from build123d import *

# Parameters (mm, degrees)
SKETCH1_W               = 25.4
SKETCH1_H               = 25.4
BOSS_EXTRUDE1_DEPTH     = 25.4
SKETCH2_W               = 22.4536
SKETCH2_H               = 20.447
CUT_EXTRUDE1_DEPTH      = 25.055020349
CUT_EXTRUDE2_DEPTH      = 32.108519733
CUT_EXTRUDE2_DEPTH_BACK = 32.108519733
SKETCH3_R               = 8.89
SKETCH4_R               = 63.5
SKETCH4_R_2             = 11.43
CUT_EXTRUDE3_DEPTH      = 26.814448745
FILLET1_R               = 1.27
FILLET2_R               = 1.27
FILLET3_R               = 0.254


with BuildPart() as part:
    # Sketch1 → Boss-Extrude1 (new body)
    with BuildSketch(Plane.XY):
        Rectangle(SKETCH1_W, SKETCH1_H)
    extrude(amount=-BOSS_EXTRUDE1_DEPTH)

    # Sketch2 → Cut-Extrude1 (cut, through all)
    with BuildSketch(Plane.XY.offset(-9.398)):
        Rectangle(SKETCH2_W, SKETCH2_H)
    extrude(amount=-CUT_EXTRUDE1_DEPTH, mode=Mode.SUBTRACT)

    # Sketch3 → Cut-Extrude2 (cut, two sides: drawn at the far end of the back side and taken through both)
    with BuildSketch(Plane.XY.offset(-CUT_EXTRUDE2_DEPTH_BACK)):
        Circle(SKETCH3_R)
    extrude(amount=CUT_EXTRUDE2_DEPTH + CUT_EXTRUDE2_DEPTH_BACK, mode=Mode.SUBTRACT)

    # Sketch4 → Cut-Extrude3 (cut, through all)
    with BuildSketch(Plane.XY.offset(-6.858)):
        Circle(SKETCH4_R)
        Circle(SKETCH4_R_2, mode=Mode.SUBTRACT)
    extrude(amount=CUT_EXTRUDE3_DEPTH, mode=Mode.SUBTRACT)

    # Fillet1
    fillet1_edges = [part.edges().sort_by_distance(p)[0] for p in [
        (-11.2268, 0, -9.398),
        (0, -10.2235, -9.398),
        (11.2268, 0, -9.398),
        (0, 10.2235, -9.398),
    ]]
    fillet(fillet1_edges, radius=FILLET1_R)

    # Fillet2
    # the kernel refuses this fillet: 1.27 mm, written as the material it adds along each edge
    with BuildSketch(Plane(origin=(-9.9568, 8.9535, -10.668), x_dir=(-1, 0, 0), z_dir=(0, 1, 0))) as fillet2_piece_1_section:
        Polygon((0, 0), (FILLET2_R, 0), (FILLET2_R, FILLET2_R), (0, FILLET2_R), align=None)
    fillet2_piece_1 = extrude(amount=FILLET2_R, mode=Mode.PRIVATE)
    fillet2_piece_1 = fillet2_piece_1 - Plane(origin=(-9.9568, 8.9535, -10.668), x_dir=(0.7071067811865475, 0, -0.7071067811865475), z_dir=(0, 1, 0)) * Sphere(FILLET2_R, mode=Mode.PRIVATE)
    add(fillet2_piece_1)
    with BuildSketch(Plane(origin=(9.9568, 8.9535, -10.668), x_dir=(0, 1, 0), z_dir=(1, 0, 0))) as fillet2_piece_2_section:
        Polygon((0, 0), (FILLET2_R, 0), (FILLET2_R, FILLET2_R), (0, FILLET2_R), align=None)
    fillet2_piece_2 = extrude(amount=FILLET2_R, mode=Mode.PRIVATE)
    fillet2_piece_2 = fillet2_piece_2 - Plane(origin=(9.9568, 8.9535, -10.668), x_dir=(0, -0.7071067811865475, -0.7071067811865475), z_dir=(1, 0, 0)) * Sphere(FILLET2_R, mode=Mode.PRIVATE)
    add(fillet2_piece_2)
    with BuildSketch(Plane(origin=(-9.9568, -8.9535, -10.668), x_dir=(-1, 0, 0), z_dir=(0, -1, 0))) as fillet2_piece_3_section:
        Polygon((0, 0), (FILLET2_R, 0), (FILLET2_R, -FILLET2_R), (0, -FILLET2_R), align=None)
    fillet2_piece_3 = extrude(amount=FILLET2_R, mode=Mode.PRIVATE)
    fillet2_piece_3 = fillet2_piece_3 - Plane(origin=(-9.9568, -8.9535, -10.668), x_dir=(0.7071067811865475, 0, -0.7071067811865475), z_dir=(0, -1, 0)) * Sphere(FILLET2_R, mode=Mode.PRIVATE)
    add(fillet2_piece_3)
    with BuildSketch(Plane(origin=(9.9568, -8.9535, -10.668), x_dir=(0, -1, 0), z_dir=(1, 0, 0))) as fillet2_piece_4_section:
        Polygon((0, 0), (FILLET2_R, 0), (FILLET2_R, -FILLET2_R), (0, -FILLET2_R), align=None)
    fillet2_piece_4 = extrude(amount=FILLET2_R, mode=Mode.PRIVATE)
    fillet2_piece_4 = fillet2_piece_4 - Plane(origin=(9.9568, -8.9535, -10.668), x_dir=(0, 0.7071067811865475, -0.7071067811865475), z_dir=(1, 0, 0)) * Sphere(FILLET2_R, mode=Mode.PRIVATE)
    add(fillet2_piece_4)
    with BuildSketch(Plane(origin=(-11.2268, -10.2235, -10.668), x_dir=(1, 0, 0), z_dir=(0, 0, -1)), Plane(origin=(11.2268, -10.2235, -10.668), x_dir=(0, 1, 0), z_dir=(0, 0, -1))) as fillet2_piece_5:
        with BuildLine():
            CenterArc((FILLET2_R, -FILLET2_R), FILLET2_R, 90, 90)
            Line((0, -FILLET2_R), (0, 0))
            Line((0, 0), (FILLET2_R, 0))
        make_face()
    extrude(amount=14.732)
    with BuildSketch(Plane(origin=(-11.2268, 10.2235, -10.668), x_dir=(1, 0, 0), z_dir=(0, 0, -1)), Plane(origin=(11.2268, 10.2235, -10.668), x_dir=(0, -1, 0), z_dir=(0, 0, -1))) as fillet2_piece_6:
        with BuildLine():
            CenterArc((FILLET2_R, FILLET2_R), FILLET2_R, 180, 90)
            Line((0, FILLET2_R), (0, 0))
            Line((0, 0), (FILLET2_R, 0))
        make_face()
    extrude(amount=14.732)

    # Fillet3
    fillet3_edges = [part.edges().sort_by_distance(p)[0] for p in [
        (-8.89, 0, 0),
        (-8.89, 0, -9.398),
    ]]
    fillet(fillet3_edges, radius=FILLET3_R)


solid = part.part
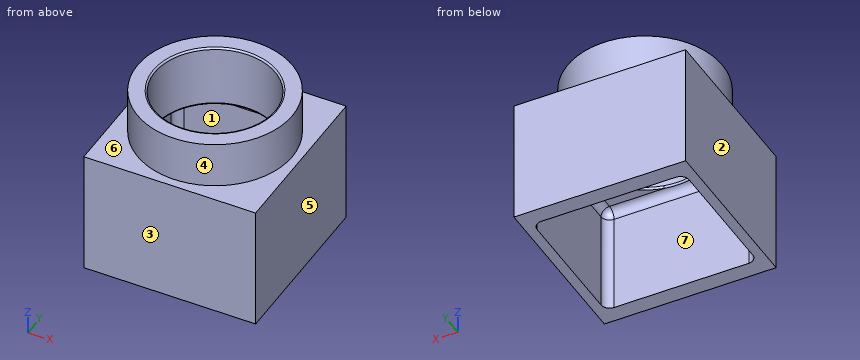
Read the model definition and answer for the solid it produces. Units are mm, in the model's axes. Face numbers are marked on the shaded views. A direction names the side the tool comes from. Coordinates: 2 decimals unless noted, no trailing zeros. Loops run counter-clockwise (first coordinate to the right, second up) from the corner with the lowest first, then second, coordinate; pieces in that order, holes last.
Q1. The part is cut by section C-C on x = 10.75. Write down the section's boundary in (y, z).
Q2. Consider probe 1 along Y at (x, z) = (0, -3.75); probe 2 along Y at (x, z) = (5.75, -18). Determine where each line is inside the solid, lowest interval first.
Q3. The part is cut by section D-D on z = -6.5. Write down the section's boundary in (x, y).
Q4. The part is cut by section A-A on y = 0. Write down the section's boundary in (x, z), and give its area (3 significant figures).
Q5. The part is cut by section B-B on z = -16.5. Write down the section's boundary in (x, y).
Q6. Each of these flat-tipped pins is pushed along its axis until it touches: pin 1 Ø1.5 at (x, z) = (1.5, -2.5) entering from -Y; pin 2 Ø14 at (x, y) = (0, 0) entering from -Z; pin 3 Ø2 at (x, y) = (2.5, -8.5) entering from -Z. Where does it stop, or does it pass through?
Q7. Which of the six approach directions +Z, -Z, +X, -X, +Y, -Y give full straight-line access (tool end or side, diameter ignored) to the marked faces 5, 6 and 7?
Q8. The mould has two halves that part along X. Classify the marked faces 1, 2, 3 and 4: +X half, -X half, draft (parallel to the pull), parting line (faces both ways), or undercut.
Results below:
1. outline: (-12.7, -25.4) - (-9.95, -25.4) - (-9.95, -10.67) arc R0.99 cw to (-8.95, -9.68) - (8.95, -9.68) arc R0.99 cw to (9.95, -10.67) - (9.95, -25.4) - (12.7, -25.4) - (12.7, -6.86) - (3.88, -6.86) - (3.88, 0) - (-3.88, 0) - (-3.88, -6.86) - (-12.7, -6.86) - close
2. probe 1: y = -11.43 to -8.89, 8.89 to 11.43
2. probe 2: y = -12.7 to -10.22, 10.22 to 12.7
3. outline: circle Ø22.86 at (0, 0); hole circle Ø17.78 at (0, 0)
4. outline: (-12.7, -25.4) - (-11.23, -25.4) - (-11.23, -10.67) arc R1.27 cw to (-9.96, -9.4) - (-9.14, -9.4) arc R0.25 ccw to (-8.89, -9.14) - (-8.89, -0.25) arc R0.25 ccw to (-9.14, 0) - (-11.43, 0) - (-11.43, -6.86) - (-12.7, -6.86) - close; (8.89, -9.14) arc R0.25 ccw to (9.14, -9.4) - (9.96, -9.4) arc R1.27 cw to (11.23, -10.67) - (11.23, -25.4) - (12.7, -25.4) - (12.7, -6.86) - (11.43, -6.86) - (11.43, 0) - (9.14, 0) arc R0.25 ccw to (8.89, -0.25) - close
4. area: 102 mm2
5. outline: (-12.7, -12.7) - (12.7, -12.7) - (12.7, 12.7) - (-12.7, 12.7) - close; hole (-11.23, -8.95) arc R1.27 ccw to (-9.96, -10.22) - (9.96, -10.22) arc R1.27 ccw to (11.23, -8.95) - (11.23, 8.95) arc R1.27 ccw to (9.96, 10.22) - (-9.96, 10.22) arc R1.27 ccw to (-11.23, 8.95) - close
6. pin 1: stops at y = -11.41
6. pin 2: passes through
6. pin 3: stops at z = -9.52
7. face 5: +Z, -Z, +X, +Y, -Y
7. face 6: +Z
7. face 7: -Z
8. face 1: undercut
8. face 2: -X half
8. face 3: draft
8. face 4: parting line
